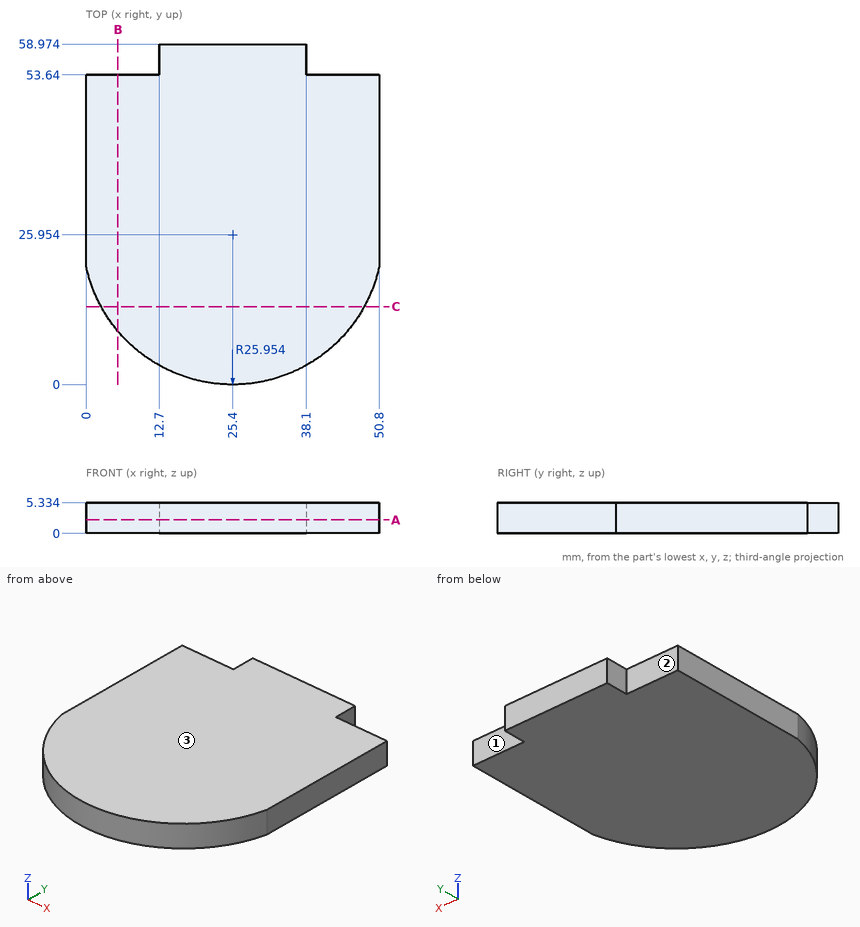
Design review of the part shown in the three views and the two pictorial views. Dimensions are in mm from the part's minimum x, y and z. A direction names the side the tool comes from. Round coordinates to 2 decimals unless told otherwise and drop trailing zeros. Write each loop counter-clockwise with the first axis right and the second up, starting at its lowest first coordinate (ties: lowest second). Pieces come first, ordered by that corner, then holes. Notation, with made-up numbers: (-36.75, -34) -> (-11.75, -34) arc R19 cw to (-11.75, -12) -> close; hole circle Ø5 at (-37.5, 13.25). An arc over 180 degrees is marked (long way). Write item = value, one per line. Start each with the question number.
1) Take a section at C-C, the plane y = 13.5. State the section outline as (x, z) points.
2) Take a section at A-A, the plane z = 2.35. State the section outline as (x, y) points, plus the area to 3 significant figures.
3) Clearance check with flat-ended pins moving along their axes: pin 1 (1.6 mm diameter, centred on x = 7, z = 1.5, fed in from +Y); pin 2 (1 mm diameter, centred on y = 18.5, z = 2, fed in from +X) (3 decimals). State where each tip first meets the part, or that it passes through.
4) Tool access review of the marked faces 1, 2 and 3: name each direction out of +Z, -Z, +X, -X, +Y, -Y from which nothing blocks a thin tool from reaching the whole face with its end or side.
5) Take a section at B-B, the plane x = 5.5. State the section outline as (y, z) points.
6) Wall thickness on probe 1 along X at (y, z) = (54.5, 4.7); probe 2 along Y at (x, z) = (40.5, 4.65); probe 3 along X at (y, z) = (8, 2.1): over which ranges is each line inside the solid? List them lowest first. Write a range as from..to.
Results list:
q1.outline = (2.63, 0) -> (48.17, 0) -> (48.17, 5.33) -> (2.63, 5.33) -> close
q2.outline = (0, 20.62) arc R25.95 ccw to (50.8, 20.62) -> (50.8, 53.64) -> (38.1, 53.64) -> (38.1, 58.97) -> (12.7, 58.97) -> (12.7, 53.64) -> (0, 53.64) -> close
q2.area = 2,600 mm²
q3.pin_1 = 53.64
q3.pin_2 = 50.405
q4.face_1 = +Z, -Z, +X, +Y
q4.face_2 = +Z, -Z, -X, +Y
q4.face_3 = +Z, +X, -X, +Y, -Y
q5.outline = (9.29, 0) -> (53.64, 0) -> (53.64, 5.33) -> (9.29, 5.33) -> close
q6.probe_1 = 12.7..38.1
q6.probe_2 = 4.84..53.64
q6.probe_3 = 6.66..44.14
